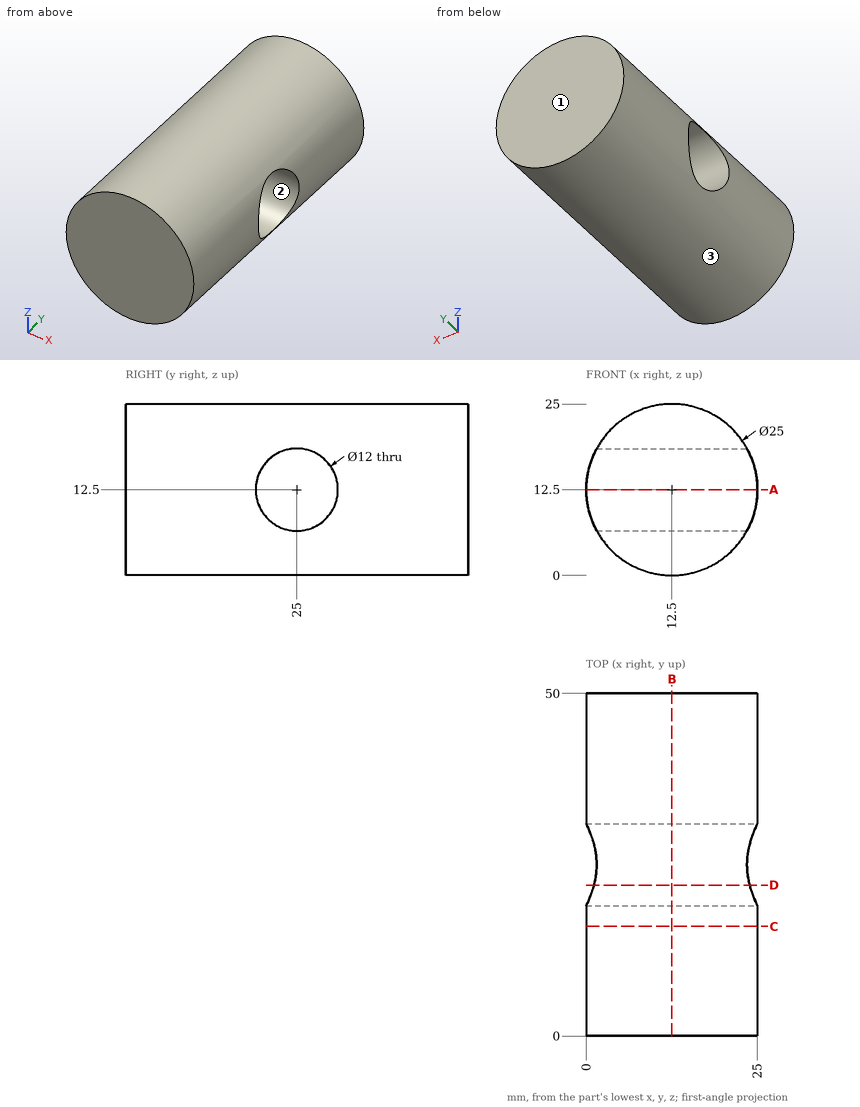
Geometry check sheet. Reference: drawing and pictorial views, mm from the part's lowest x, y, z. Coordinates: 2 decimals unless noted, no trailing zeros. Order: outer loops, then holes, each group sorted by start corner. A loop starts at its lowest first (then second) coordinate and runs counter-clockwise, first axis right, second up. Notation, with made-up numbers: (54.25, 6) -> (96.25, 6) arc R18 cw to (96.25, 11) -> close; hole circle Ø5 at (12.5, -13.5). An arc over 180 degrees is marked (long way). Write item = value, one per line. Start each with the question number.
1) Material ranges on L1, parallel to Z at x = 18.5, y = 25; L2, parallel to Y at x = 4, z = 9.5; L3, parallel to Z at x = 20, y = 25, recorded low to high.
2) Cross-section at B-B (x = 12.5). Enter the section's corners in (y, z), then the cut area to 3 significant figures.
3) Mould release check, pull along Z, two halves, no side actions. Record for the marked faces 1, 2 and 3: +Z half, -Z half, draft (parallel to the pull), parting line (faces both ways), or undercut.
4) Cross-section at A-A (z = 12.5). Enter the section's corners in (x, y).
5) Cross-section at D-D (y = 22). Enter the section's corners in (x, z), then the cut area to 3 significant figures.
6) Go/stop test with flat-tipped pins: P1, Ø10, axis at x = 20.5, y = 38, coming from the +Z side; P2, Ø10, axis at y = 21.5, z = 9, coming from the +X side; P3, Ø5, axis at x = 17, y = 29.5, coming from the +Z side; P4, Ø3, axis at x = 20.5, y = 23.5, coming from the -Z side. Record where each tip stops, or that it passes through.
7) Cross-section at C-C (y = 16). Enter the section's corners in (x, z).
Ans:
q1.L1 = 1.53 to 6.5, 18.5 to 23.47
q1.L2 = 0 to 19.8, 30.2 to 50
q1.L3 = 2.5 to 6.5, 18.5 to 22.5
q2.outline = (0, 0) -> (50, 0) -> (50, 25) -> (0, 25) -> close; hole circle Ø12 at (25, 12.5)
q2.area = 1,140 mm²
q3.face_1 = draft
q3.face_2 = undercut
q3.face_3 = parting line
q4.outline = (0, 0) -> (25, 0) -> (25, 19) -> (0, 19) -> close; (0, 31) -> (25, 31) -> (25, 50) -> (0, 50) -> close
q5.outline = (1.13, 7.3) arc R12.5 ccw to (23.87, 7.3) -> close; (1.13, 17.7) -> (23.87, 17.7) arc R12.5 ccw to start
q5.area = 239 mm²
q6.P1 = 24.63
q6.P2 = 25
q6.P3 = 24.84
q6.P4 = 1.82
q7.outline = circle Ø25 at (12.5, 12.5)
